Geometry: final body of the model. Coordinates: model frame, mm. A direction names the side the tool comes from. Give positions to 0.01 mm unless a question says otherwise; leave off trailing zeros. Write each loop counter-clockwise with the first axis right and the second up, starting at its lowest first coordinate (ties: lowest second). Pieces come first, ordered by that corner, then holes. Notation, with made-up numbers: (-0.5, 61.25) -> (8.5, 61.25) arc R20 ccw to (8.5, 91.25) -> close; hole circle Ø10 at (82, 64). An arc over 180 degrees is marked (long way). Answer in a Markdown table with one row per item. Add a question column.
Autodesk Inventor part; units mm, degrees
ref_plane "YZ Plane" through (0, 0, 0) normal (1, 0, 0) x (0, 1, 0)
ref_plane "XZ Plane" through (0, 0, 0) normal (0, 1, 0) x (-1, 0, 0)
ref_plane "XY Plane" through (0, 0, 0) normal (0, 0, 1) x (1, 0, 0)
sketch "Sketch1" plane through (0, 0, 0) normal (0, 0, 1) x (1, 0, 0)
  line L0 (-304.6106, 302.7116) -> (304.9894, 302.7116)
  line L1 (304.9894, 302.7116) -> (304.9894, -306.8884)
  line L2 (304.9894, -306.8884) -> (-304.6106, -306.8884)
  line L3 (-304.6106, -306.8884) -> (-304.6106, 302.7116)
  point P0 (0, 0)
  dimension "d0" = 609.6
  dimension "d2" = 609.6
extrude "Extrusion1" add sketch "Sketch1" along normal blind 19.05
sketch "Sketch2" plane through (0, 0, 19.05) normal (0, 0, 1) x (1, 0, 0)
  circle A0 centre (-242.6981, -160.8384) radius 4.7625
  circle A1 centre (243.0642, -160.8384) radius 4.7625
  circle A2 centre (243.0642, 156.6616) radius 4.7625
  circle A3 centre (-242.6981, 156.6616) radius 4.7625
  circle A4 centre (-157.7669, -219.5759) radius 4.7625
  circle A5 centre (158.1456, -219.5759) radius 4.7625
  circle A6 centre (158.1456, 215.3991) radius 4.7625
  circle A7 centre (-157.7669, 215.3991) radius 4.7625
  point P0 (-304.6106, -306.8884)
  point P1 (0, 0)
  point P2 (304.9894, 302.7116)
  point P3 (-304.6106, 302.7116)
  point P4 (304.9894, -306.8884)
  dimension "d5" = 9.525
  dimension "d6" = 146.05
  dimension "d7" = 61.9125
  dimension "d15" = 9.525
  dimension "d16" = 146.05
  dimension "d17" = 61.9252
  dimension "d18" = 9.525
  dimension "d19" = 61.9252
  dimension "d20" = 146.05
  dimension "d21" = 9.525
  dimension "d22" = 61.9125
  dimension "d23" = 146.05
  dimension "d24" = 9.525
  dimension "d25" = 146.8438
  dimension "d26" = 87.3125
  dimension "d27" = 9.525
  dimension "d28" = 146.8438
  dimension "d29" = 87.3125
  dimension "d30" = 9.525
  dimension "d31" = 87.3125
  dimension "d32" = 146.8438
  dimension "d33" = 9.525
  dimension "d34" = 146.8438
  dimension "d35" = 87.3125
hole "Hole2" at (-242.6981, -160.8384, 19.05) at (-242.6981, 156.6616, 19.05) at (-157.7669, 215.3991, 19.05) at (158.1456, 215.3991, 19.05) at (243.0642, 156.6616, 19.05) at (243.0642, -160.8384, 19.05) at (158.1456, -219.5759, 19.05) at (-157.7669, -219.5759, 19.05) direction (0, 0, -1) diameter 9.525 end through all counterbore diameter 25.4 counterbore depth 4.7625
sketch "Sketch3" plane through (0, 0, 19.05) normal (0, 0, 1) x (1, 0, 0)
  line L0 (-117.475, -85.725) -> (117.475, -85.725)
  line L1 (117.475, -85.725) -> (117.475, 85.725)
  line L2 (117.475, 85.725) -> (-117.475, 85.725)
  line L3 (-117.475, 85.725) -> (-117.475, -85.725)
  line L4 (-117.475, -85.725) -> (117.475, 85.725) construction
  line L5 (117.475, -85.725) -> (-117.475, 85.725) construction
  point P0 (0, 0)
  dimension "d43" = 234.95
  dimension "d44" = 171.45
extrude "Extrusion2" cut sketch "Sketch3" against normal blind 19.05
sketch "Sketch4" plane through (0, 0, 19.05) normal (0, 0, 1) x (1, 0, 0)
  line L0 (117.475, 85.725) -> (117.475, -85.725)
  line L1 (117.475, -85.725) -> (-117.475, -85.725)
  line L2 (-117.475, -85.725) -> (-117.475, 85.725)
  line L3 (-117.475, 85.725) -> (117.475, 85.725)
  arc A0 (-107.95, 95.25) -> (-127, 76.2) centre (-107.95, 76.2) ccw
  line L4 (-107.95, 76.2) -> (-107.95, 95.25) construction
  line L5 (-107.95, 76.2) -> (-88.9, 76.2) construction
  line L6 (-107.95, 76.2) -> (-127, 76.2) construction
  arc A1 (-127, -80.1017) -> (-108.2751, -95.25) centre (-108.2751, -76.1028) ccw
  arc A2 (108.1693, -95.25) -> (127, -75.9762) centre (107.9478, -76.1978) ccw
  line L7 (107.9478, -76.1978) -> (127, -75.9762) construction
  line L8 (107.9478, -76.1978) -> (108.1693, -95.25) construction
  arc A3 (127, 76.5685) -> (108.3185, 95.25) centre (108.3185, 76.5685) ccw
  line L9 (127, -75.9762) -> (127, 76.5685)
  line L10 (-107.95, 95.25) -> (108.3185, 95.25)
  line L11 (108.1693, -95.25) -> (-108.2751, -95.25)
  line L12 (-127, 76.2) -> (-127, -80.1017)
  point P0 (0, 0)
  dimension "d47" = 19.05
  dimension "d48" = 90
  dimension "d49" = 90
  dimension "d50" = 9.525
  dimension "d51" = 9.525
  dimension "d52" = 9.525
  dimension "d53" = 9.525
  dimension "d54" = 90
  dimension "d55" = 9.525
  dimension "d56" = 9.525
  dimension "d57" = 9.525
  dimension "d58" = 9.525
extrude "Extrusion3" cut sketch "Sketch4" against normal blind 6.35
sketch "Sketch5" plane through (0, 0, 19.05) normal (0, 0, 1) x (1, 0, 0)
  line L0 (-304.6106, 302.7116) -> (-304.6106, -306.8884)
  line L1 (-304.6106, -306.8884) -> (304.9894, -306.8884)
  line L2 (304.9894, -306.8884) -> (304.9894, 302.7116)
  line L3 (-212.5356, 306.8884) -> (-193.4856, 306.8884)
  line L4 (-193.4856, 306.8884) -> (-193.4856, -306.8884)
  line L5 (-193.4856, -306.8884) -> (-212.5356, -306.8884)
  line L6 (-212.5356, -306.8884) -> (-212.5356, 306.8884)
  line L7 (-212.5356, 306.8884) -> (-193.4856, -306.8884) construction
  line L8 (-193.4856, 306.8884) -> (-212.5356, -306.8884) construction
  line L9 (193.8644, 306.8884) -> (212.9144, 306.8884)
  line L10 (212.9144, 306.8884) -> (212.9144, -306.8884)
  line L11 (212.9144, -306.8884) -> (193.8644, -306.8884)
  line L12 (193.8644, -306.8884) -> (193.8644, 306.8884)
  line L13 (193.8644, 306.8884) -> (212.9144, -306.8884) construction
  line L14 (212.9144, 306.8884) -> (193.8644, -306.8884) construction
  point P0 (0, 0)
  point P1 (-203.0106, 0)
  point P2 (203.3894, 0)
  dimension "d61" = 19.05
  dimension "d62" = 101.6
  dimension "d63" = 19.05
  dimension "d64" = 101.6
extrude "Extrusion4" cut sketch "Sketch5" against normal blind 9.525
properties part number "router_table_1"
Q1. Section C-C on z = 5.5. Count the separate pieces of the cut face and the enclosed holes in it, and give its area (3 significant figures).
Q2. Section A-A on y = -2.5. Return loops of the section in (x, z) (3 decimals), and give its area (3 significant figures).
Q3. Contact query for a flat-ended pin moving along its axis: pin 1 Ø7.5 at (x, y) = (246, 159.5) entering from +Z. Output: stop coordinate, or through.
Q4. Pull-direction query (Y, two-part tool) for faces 1 (the flat face through (-4, 302.712, 9)), 2 (the flat face through (203, 2, 9.525)), 3 (the cylindrical face through (232.36, 149.83, 16.64)); classes: +Y half, -Y half, draft (parallel to the pull), parting line (faces both ways), or undercut.
Q5. Section B-B on x = -86.5. Return loops of the section in (y, z) (3 decimals).
Q6. Line query: probe 1 along X at (y, z) = (-260, 15); probe 2 along X at (y, z) = (58, 3) (3 decimals); probe 3 along Y at (x, z) = (-40, 14.25). Output: solid intervals per line, ascending. Write a range as from..to.
Q7. Section D-D on y = -136.5. Return loops of the section in (x, z) (3 decimals).
Q8. Access query for faces 4 (the flat face through (-203, 2, 9.525)), 5 (the cylindrical face through (-120.46, -90.87, 15.92)), 6 (the flat face through (-259, 2, 19.05)). Directions: +Z, -Z, +X, -X, +Y, -Y. A direction counts if a zero-diameter tool reaches every point of the face in a straight line with its end or side. Return the directions, or none.
Checks:
| question | item | result |
|---|---|---|
| 1 | separate pieces | 1 |
| 1 | enclosed holes | 9 |
| 1 | area | 331,000 mm^2 |
| 2 | outline | (-304.611, 0) -> (-117.475, 0) -> (-117.475, 12.7) -> (-127, 12.7) -> (-127, 19.05) -> (-193.486, 19.05) -> (-193.486, 9.525) -> (-212.536, 9.525) -> (-212.536, 19.05) -> (-304.611, 19.05) -> close; (117.475, 0) -> (304.989, 0) -> (304.989, 19.05) -> (212.914, 19.05) -> (212.914, 9.525) -> (193.864, 9.525) -> (193.864, 19.05) -> (127, 19.05) -> (127, 12.7) -> (117.475, 12.7) -> close |
| 2 | area | 6,650 mm^2 |
| 3 | pin 1 | z = 14.29 |
| 4 | face 1 | +Y half |
| 4 | face 2 | draft |
| 4 | face 3 | undercut |
| 5 | outline | (-306.888, 0) -> (-85.725, 0) -> (-85.725, 12.7) -> (-95.25, 12.7) -> (-95.25, 19.05) -> (-306.888, 19.05) -> close; (85.725, 0) -> (302.712, 0) -> (302.712, 19.05) -> (95.25, 19.05) -> (95.25, 12.7) -> (85.725, 12.7) -> close |
| 6 | probe 1 | -304.61..-212.54, -193.49..193.86, 212.91..304.99 |
| 6 | probe 2 | -304.611..-117.475, 117.475..304.989 |
| 6 | probe 3 | -306.89..-95.25, 95.25..302.71 |
| 7 | outline | (-304.611, 0) -> (304.989, 0) -> (304.989, 19.05) -> (212.914, 19.05) -> (212.914, 9.525) -> (193.864, 9.525) -> (193.864, 19.05) -> (-193.486, 19.05) -> (-193.486, 9.525) -> (-212.536, 9.525) -> (-212.536, 19.05) -> (-304.611, 19.05) -> close |
| 8 | face 4 | +Z, +Y, -Y |
| 8 | face 5 | +Z |
| 8 | face 6 | +Z, +X, -X, +Y, -Y |
